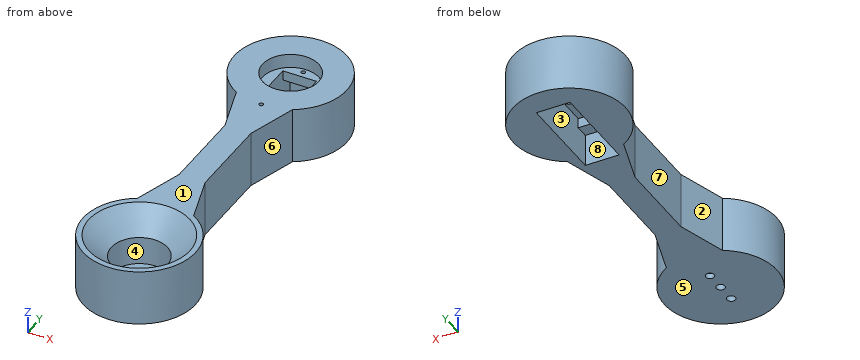
Autodesk Inventor part; units mm, degrees
ref_plane "YZ Plane" through (0, 0, 0) normal (1, 0, 0) x (0, 1, 0)
ref_plane "XZ Plane" through (0, 0, 0) normal (0, 1, 0) x (-1, 0, 0)
ref_plane "XY Plane" through (0, 0, 0) normal (0, 0, 1) x (1, 0, 0)
sketch "Sketch1" plane through (0, 0, 0) normal (0, 0, 1) x (1, 0, 0)
  circle A0 centre (0, 0) radius 10
  circle A1 centre (0, 0) radius 30
  line L0 (0, 0) -> (10, 0)
  line L1 (10, 0) -> (10, 100)
  line L2 (10, 100) -> (0, 100)
  line L3 (0, 100) -> (0, 0)
  line L4 (0, 100) -> (-10, 100)
  line L5 (-10, 100) -> (-10, 0)
  line L6 (-10, 0) -> (0, 0)
  line L7 (0, 0) -> (0, 100)
  circle A2 centre (0, 100) radius 30
  circle A3 centre (0, 100) radius 10
  circle A4 centre (0, 0) radius 20
  circle A5 centre (0, 100) radius 20
  point P0 (10, 17.3205)
  point P1 (10, 82.6795)
  point P2 (-10, 82.6795)
  point P3 (-10, 17.3205)
  dimension "d0" = 20
  dimension "d1" = 60
  dimension "d2" = 10
  dimension "d3" = 100
  dimension "d4" = 60
  dimension "d5" = 40
  dimension "d6" = 40
extrude "Extrusion1" add sketch "Sketch1" along normal blind 20 contours L5 A4 L3 A0 | A0 L1 A4 L5 | A0 L3 A4 L1 | L5 A1 L3 A4 | A4 L3 A1 L1 | L5 A2 L3 A1 | A1 L3 A2 L1 | L5 A5 L3 A2 | A2 L3 A5 L1 | A5 L1 A3 L5 | L5 A3 L3 A5 | A5 L3 A3 L1 | A3 L2 L4 | L4 L3 A3 | A3 L3 L2
sketch "Sketch2" plane through (0, 0, 20) normal (0, 0, 1) x (1, 0, 0)
  circle A0 centre (0, 100) radius 10
  point P0 (0, 0)
  dimension "d9" = 20
extrude "Extrusion2" cut sketch "Sketch2" against normal blind 5
sketch "Sketch3" plane through (0, 0, 0) normal (0, 0, -1) x (-1, 0, 0)
  line L0 (0, 100) -> (6, 100)
  line L1 (6, 100) -> (6, 83)
  line L2 (6, 83) -> (0, 83)
  line L3 (0, 83) -> (0, 100)
  line L4 (0, 100) -> (-6, 100)
  line L5 (-6, 100) -> (-6, 83)
  line L6 (-6, 83) -> (0, 83)
  line L7 (0, 83) -> (0, 100)
  line L8 (6, 100) -> (-6, 100)
  line L9 (-6, 100) -> (-6, 106)
  line L10 (-6, 106) -> (6, 106)
  line L11 (6, 106) -> (6, 100)
  point P0 (0, 0)
  dimension "d12" = 6
  dimension "d13" = 17
  dimension "d14" = 6
  dimension "d15" = 6
extrude "Extrusion3" cut sketch "Sketch3" against normal blind 15
sketch "Sketch4" plane through (0, 0, 0) normal (0, 0, -1) x (-1, 0, 0)
  line L0 (6, 83) -> (-6, 83)
  line L1 (-6, 83) -> (-6, 78.3)
  line L2 (-6, 78.3) -> (6, 78.3)
  line L3 (6, 78.3) -> (6, 83)
  line L4 (6, 106) -> (-6, 106)
  line L5 (6, 106) -> (-6, 106)
  line L6 (-6, 106) -> (-6, 110.7)
  line L7 (-6, 110.7) -> (6, 110.7)
  line L8 (6, 110.7) -> (6, 106)
  point P0 (0, 0)
  dimension "d18" = 12
  dimension "d19" = 4.7
  dimension "d20" = 4.7
extrude "Extrusion4" cut sketch "Sketch4" against normal blind 11.5
sketch "Sketch5" plane through (0, 0, 11.5) normal (0, 0, -1) x (-1, 0, 0)
  line L0 (6, 110.7) -> (6, 78.3)
  line L1 (-6, 78.3) -> (-6, 110.7)
  line L2 (6, 110.7) -> (-6, 110.7)
  line L3 (-6, 110.7) -> (-6, 108.4)
  line L4 (-6, 108.4) -> (6, 108.4)
  line L5 (6, 108.4) -> (6, 110.7)
  line L6 (6, 78.2245) -> (-6, 78.2245)
  line L7 (-6, 78.2245) -> (-6, 80.5245)
  line L8 (-6, 80.5245) -> (6, 80.5245)
  line L9 (6, 80.5245) -> (6, 78.2245)
  circle A0 centre (0, 108.4) radius 0.75
  circle A1 centre (0, 80.5245) radius 0.75
  point P0 (0, 0)
  dimension "d23" = 2.3
  dimension "d24" = 2.3
  dimension "d25" = 1.5
  dimension "d26" = 1.5
extrude "Extrusion5" cut sketch "Sketch5" against normal blind 48.975 contours A0 L4 | L4 A0 | A1 L8 | L8 A1
sketch "Sketch6" plane through (0, 0, 0) normal (0, 0, -1) x (-1, 0, 0)
  circle A0 centre (0, 0) radius 10
extrude "Extrusion6" add sketch "Sketch6" against normal blind 2
sketch "Sketch7" plane through (0, 0, 0) normal (0, 0, -1) x (-1, 0, 0)
  circle A0 centre (0, 0) radius 1.5
  circle A1 centre (0, 7) radius 1.5
  circle A2 centre (0, -7) radius 1.5
  dimension "d31" = 3
  dimension "d32" = 3
  dimension "d33" = 3
extrude "Extrusion7" cut sketch "Sketch7" against normal blind 10.7
chamfer "Chamfer1" distance 8 angle 45 1 edges at (-10, 0, 20)
sketch "Sketch8" plane through (0, 0, 20) normal (0, 0, 1) x (1, 0, 0)
  line L0 (-10, 82.6795) -> (-10, 17.3205)
  line L1 (10, 17.3205) -> (10, 82.6795)
  line L2 (-10, 82.6795) -> (10, 17.3205)
  line L3 (10, 17.3205) -> (10, 82.6795)
  arc A0 (-10, 17.3205) -> (10, 17.3205) centre (0, 0) ccw
  line L4 (10, 82.6795) -> (-10, 17.3205)
  line L5 (-10, 17.3205) -> (-10, 82.6795)
  line L6 (0, 50) -> (4.6328, 50)
  line L7 (4.6328, 50) -> (4.6328, 65.1396)
  line L8 (4.6328, 65.1396) -> (0, 65.1396)
  line L9 (0, 65.1396) -> (0, 50)
  line L10 (0, 50) -> (4.6328, 50)
  line L11 (4.6328, 50) -> (4.6328, 34.8604)
  line L12 (4.6328, 34.8604) -> (0, 34.8604)
  line L13 (0, 34.8604) -> (0, 50)
  line L14 (4.6328, 34.8604) -> (-4.6328, 34.8604)
  line L15 (-4.6328, 34.8604) -> (-4.6328, 65.1396)
  line L16 (-4.6328, 65.1396) -> (4.6328, 65.1396)
  line L17 (4.6328, 65.1396) -> (4.6328, 34.8604)
extrude "Extrusion8" cut sketch "Sketch8" against normal blind 38.5125 contours L2 L15 L4 L0 | L2 L11 L7 L4 L1
properties part number "2nd arm"
Design review of the part built by this model. Coordinates are the model's own, in mm. Face numbers are marked on the shaded views. A direction names the side the tool comes from. Round coordinates to 2 decimals unless told otherwise and drop trailing zeros. Write each loop counter-clockwise with the first axis right and the second up, starting at its lowest first coordinate (ties: lowest second). Pieces come first, ordered by that corner, then holes. Notation, with made-up numbers: (-25.75, 60.5) - (9.25, 60.5) arc R18 ccw to (9.25, 85.5) - close; hole circle Ø5 at (63.25, -36.75). An arc over 180 degrees is marked (long way). Use a Markdown table: item, result. Add a question column.
1. Mouldability with a two-part tool opening along X and no side actions: class the marked faces 1, 2 and 3 as +X half, -X half, draft (parallel to the pull), parting line (faces both ways), or undercut.
2. Wall thickness on probe 1 along Y at (x, z) = (0, 1.2); probe 2 along Y at (x, z) = (0, 14.25); probe 3 along Y at (x, z) = (0, 17.5): over which ranges is each line inside the solid? List them lowest first.
3. We need section B-B (z = 6). State the section outline as (x, y) points, then the cut area to 3 significant figures.
4. We need section C-C (y = 96.5). State the section outline as (x, z) points.
5. For the marked faces 4, 5, 6, 7 and 8, list the 3-axis set-ups (+Z, -Z, +X, -X, +Y, -Y) from which the entire face can be reached by the end or side of a thin tool; tool diameter is ignored.
6. We need section A-A (y = 0). State the section outline as (x, z) points.
7. Clearance check with flat-ended pins moving along their axes: pin 1 (1 mm diameter, centred on x = -0.5, z = 12.5, fed in from -Y); pin 2 (2 mm diameter, centred on x = 0, y = 108.4, fed in from +Z); pin 3 (4 mm diameter, centred on x = 1.5, y = 81, fed in from -Z); pin 4 (2 mm diameter, centred on x = -16, y = 84.5, fed in from +Z). State where each tip first meets the part, or that it passes through.
Output:
| question | item | result |
|---|---|---|
| 1 | face 1 | draft |
| 1 | face 2 | -X half |
| 1 | face 3 | undercut |
| 2 | probe 1 | y = -20 to -8.5, -5.5 to -1.5, 1.5 to 5.5, 8.5 to 78.3, 110.7 to 120 |
| 2 | probe 2 | y = -20 to -12.25, 12.25 to 79.77, 81.27 to 83, 106 to 107.65, 109.15 to 120 |
| 2 | probe 3 | y = -20 to -15.5, 15.5 to 79.77, 81.27 to 90, 110 to 120 |
| 3 | outline | (-10, 17.32) arc R20 ccw (long way) to (10, 17.32) - (4.63, 34.86) - (4.63, 65.14) - (10, 82.68) arc R20 ccw (long way) to (-10, 82.68) - (-4.63, 65.14) - (-4.63, 34.86) - close; hole circle Ø20 at (0, 0); hole (-6, 78.3) - (6, 78.3) - (6, 110.7) - (-6, 110.7) - close |
| 3 | area | 2,530 mm2 |
| 4 | outline | (-19.69, 0) - (-6, 0) - (-6, 15) - (-9.37, 15) - (-9.37, 20) - (-19.69, 20) - close; (6, 0) - (19.69, 0) - (19.69, 20) - (9.37, 20) - (9.37, 15) - (6, 15) - close |
| 5 | face 4 | +Z |
| 5 | face 5 | -Z, +X, -X, +Y, -Y |
| 5 | face 6 | +Z, -Z, +X |
| 5 | face 7 | +Z, -Z, -X |
| 5 | face 8 | -Z |
| 6 | outline | (-20, 0) - (-1.5, 0) - (-1.5, 2) - (-10, 2) - (-10, 12) - (-18, 20) - (-20, 20) - close; (1.5, 0) - (20, 0) - (20, 20) - (18, 20) - (10, 12) - (10, 2) - (1.5, 2) - close |
| 7 | pin 1 | stops at y = -20 |
| 7 | pin 2 | stops at z = 15 |
| 7 | pin 3 | stops at z = 11.5 |
| 7 | pin 4 | passes through |
